Autodesk Inventor part; units mm, degrees
ref_plane "YZ Plane" through (0, 0, 0) normal (1, 0, 0) x (0, 1, 0)
ref_plane "XZ Plane" through (0, 0, 0) normal (0, 1, 0) x (-1, 0, 0)
ref_plane "XY Plane" through (0, 0, 0) normal (0, 0, 1) x (1, 0, 0)
sketch "Sketch1" plane through (0, 0, 0) normal (0, 1, 0) x (-1, 0, 0)
  line L0 (200, 0) -> (-200, 0)
  line L1 (200, 0) -> (750, 550)
  line L2 (750, 550) -> (750, 1150)
  line L3 (750, 1150) -> (-750, 1150)
  line L4 (-750, 1150) -> (-750, 550)
  line L5 (-750, 550) -> (-200, 0)
  point P0 (0, 0)
  point P1 (0, 0)
  point P2 (0, 1150)
  dimension "d0" = 400
  dimension "d1" = 1150
  dimension "d2" = 600
  dimension "d3" = 1500
extrude "Extrusion1" add sketch "Sketch1" along normal blind 450
properties part number "DUMMY 2"
For this review, take the finished solid that the model builds, in its own axes (mm). Round coordinates to 2 decimals unless told otherwise and drop trailing zeros. Write each loop counter-clockwise with the first axis right and the second up, starting at its lowest first coordinate (ties: lowest second). Pieces come first, ordered by that corner, then holes. Notation, with made-up numbers: (-6.75, -36.75) - (45.25, -36.75) arc R20 cw to (45.25, -30.75) - close; hole circle Ø3 at (19, -35). An arc over 180 degrees is marked (long way). Put each result on its own line as item: value.
Q1. We need section A-A (y = 200). Give the boundary of the cut face in (x, z).
Solved:
outline: (-750, 550) - (-200, 0) - (200, 0) - (750, 550) - (750, 1150) - (-750, 1150) - close
Q2. Wall thickness on probe 1 along X at (y, z) = (362, 443); probe 2 along Z at (x, y) = (553.5, 209.5); probe 3 along Z at (x, y) = (535.5, 276.5): over which ranges is each line inside the solid? List them lowest first.
Solved:
probe 1: x = -643 to 643
probe 2: z = 353.5 to 1150
probe 3: z = 335.5 to 1150
Q3. We need section C-C (z = 241). Give the boundary of the cut face in (x, y).
Solved:
outline: (-441, 0) - (441, 0) - (441, 450) - (-441, 450) - close
Q4. We need section B-B (x = 583). Give the boundary of the cut face in (y, z), and give its area (3 significant figures).
Solved:
outline: (0, 383) - (450, 383) - (450, 1150) - (0, 1150) - close
area: 345,000 mm2
Q5. Insertion check: pin 1 Ø12 at (y, z) = (304.5, 277.5) entering from +X. The pin has a flat end and moves straight along its axis. Give the tip position at first contact, or say it passes through.
Solved:
pin 1: stops at x = 483.5
